Input: part model. Units: mm. Frame: model coordinates. Face numbers are marked on the shaded views. Give positions to 0.01 mm unless a question says otherwise; leave off trailing zeros. Loops run counter-clockwise (first coordinate to the right, second up) from the corner with the lowest first, then second, coordinate; pieces in that order, holes last. Notation, with made-up numbers: (46, -18) -> (82, -18) arc R26 ccw to (82, 2) -> close; hole circle Ø2 at (71.25, -26.5). An arc over 180 degrees is marked (long way). Answer as a JSON object with one key per item and string values. Group by question number.
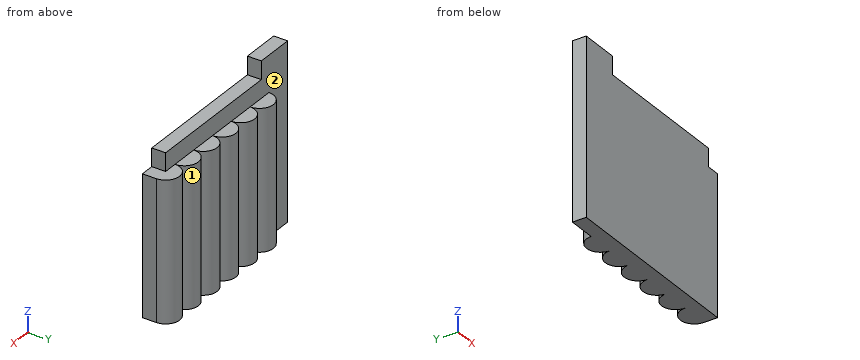
```python
from build123d import *

# Parameters (mm, degrees)
F1_DEPTH = 50
F2_W     = 70
F2_H     = 5
F3_DEPTH = 6.5
F5_W     = 5
F5_H     = 6.5
F6_DEPTH = 5
F4_W     = 14
F4_H     = 5
F7_DEPTH = 6.5


with BuildPart() as f1:
    # F0 (on Top) → F1 (new body)
    with BuildSketch(Plane.XY):
        with BuildLine():
            Line((-32.032276, 5), (-32.032276, 0))
            Line((-32.032276, 0), (37.967724, 0))
            Line((37.967724, 0), (37.967724, 5))
            ThreePointArc((37.967724, 5), (32.967724, 10), (27.967724, 5))
            ThreePointArc((27.967724, 5), (22.967724, 10), (17.967724, 5))
            ThreePointArc((17.967724, 5), (12.967724, 10), (7.967724, 5))
            ThreePointArc((7.967724, 5), (2.967724, 10), (-2.032276, 5))
            ThreePointArc((-2.032276, 5), (-7.032276, 10), (-12.032276, 5))
            ThreePointArc((-12.032276, 5), (-17.032276, 10), (-22.032276, 5))
            Line((-22.032276, 5), (-32.032276, 5))
        make_face()
    extrude(amount=F1_DEPTH)

    # F2 (on face) → F3 (join)
    with BuildSketch(Plane.XY.offset(50)):
        with Locations((2.967724, 2.5)):
            Rectangle(F2_W, F2_H)
    extrude(amount=F3_DEPTH)

    # F5 (on face) → F6 (cut)
    with BuildSketch(Plane.YZ.offset(37.967724)):
        with Locations((2.5, 53.25)):
            Rectangle(F5_W, F5_H)
    extrude(amount=-F6_DEPTH, mode=Mode.SUBTRACT)

    # F4 (on face) → F7 (join)
    with BuildSketch(Plane.XY.offset(56.5)):
        with Locations((-25.032276, 2.5)):
            Rectangle(F4_W, F4_H)
    extrude(amount=F7_DEPTH)


solid = f1.part
```
Q1. Pin query (flat end, axial travel): pin 1 Ø1 at (x, z) = (18.5, 11.5) entering from +Y; pin 2 Ø5 at (y, z) = (5.5, 36.5) entering from +X; pin 3 Ø2.5 at (x, y) = (-19, 8.5) entering from +Z; pin 4 Ø5.5 at (x, y) = (14, 7) entering from +Z. Return the tip coordinate at first contact, or that it passes through.
Q2. Section D-D on z = 58. Return the cut outline in (x, y).
Q3. Section C-C on y = 2.25. Return the cut outline in (x, z).
Q4. Section A-A on y = 6.5. Return the cut outline in (x, z), then the cut area to 3 significant figures.
Q5. Ray query, probe 1 along X at (y, z) = (8, 32); probe 2 along X at (y, z) = (7, 26); probe 3 along Z at (x, y) = (34, 9.75). Return the intervals inside material, ascending.
Q6. Section B-B on z = 36. Return the cut outline in (x, y), then the cut area to 3 significant figures.
Q7. Pull-direction query (X, two-part tool) for the marked faces 1 and 2; classes: +X half, -X half, draft (parallel to the pull), parting line (faces both ways), or undercut.
Numbers:
{
 "1": {"pin 1": "stops at y = 8.04", "pin 2": "stops at x = 37.97", "pin 3": "stops at z = 50", "pin 4": "stops at z = 56.5"},
 "2": {"outline": "(-32.03, 0) -> (-18.03, 0) -> (-18.03, 5) -> (-32.03, 5) -> close"},
 "3": {"outline": "(-32.03, 0) -> (37.97, 0) -> (37.97, 50) -> (32.97, 50) -> (32.97, 56.5) -> (-18.03, 56.5) -> (-18.03, 63) -> (-32.03, 63) -> close"},
 "4": {"outline": "(-21.8, 0) -> (-12.26, 0) -> (-12.26, 50) -> (-21.8, 50) -> close; (-11.8, 0) -> (-2.26, 0) -> (-2.26, 50) -> (-11.8, 50) -> close; (-1.8, 0) -> (7.74, 0) -> (7.74, 50) -> (-1.8, 50) -> close; (8.2, 0) -> (17.74, 0) -> (17.74, 50) -> (8.2, 50) -> close; (18.2, 0) -> (27.74, 0) -> (27.74, 50) -> (18.2, 50) -> close; (28.2, 0) -> (37.74, 0) -> (37.74, 50) -> (28.2, 50) -> close", "area": "2,860 mm²"},
 "5": {"probe 1": "x = -21.03 to -13.03, -11.03 to -3.03, -1.03 to 6.97, 8.97 to 16.97, 18.97 to 26.97, 28.97 to 36.97", "probe 2": "x = -21.61 to -12.45, -11.61 to -2.45, -1.61 to 7.55, 8.39 to 17.55, 18.39 to 27.55, 28.39 to 37.55", "probe 3": "z = 0 to 50"},
 "6": {"outline": "(-32.03, 0) -> (37.97, 0) -> (37.97, 5) arc R5 ccw to (27.97, 5) arc R5 ccw to (17.97, 5) arc R5 ccw to (7.97, 5) arc R5 ccw to (-2.03, 5) arc R5 ccw to (-12.03, 5) arc R5 ccw to (-22.03, 5) -> (-32.03, 5) -> close", "area": "586 mm²"},
 "7": {"face 1": "undercut", "face 2": "draft"}
}
